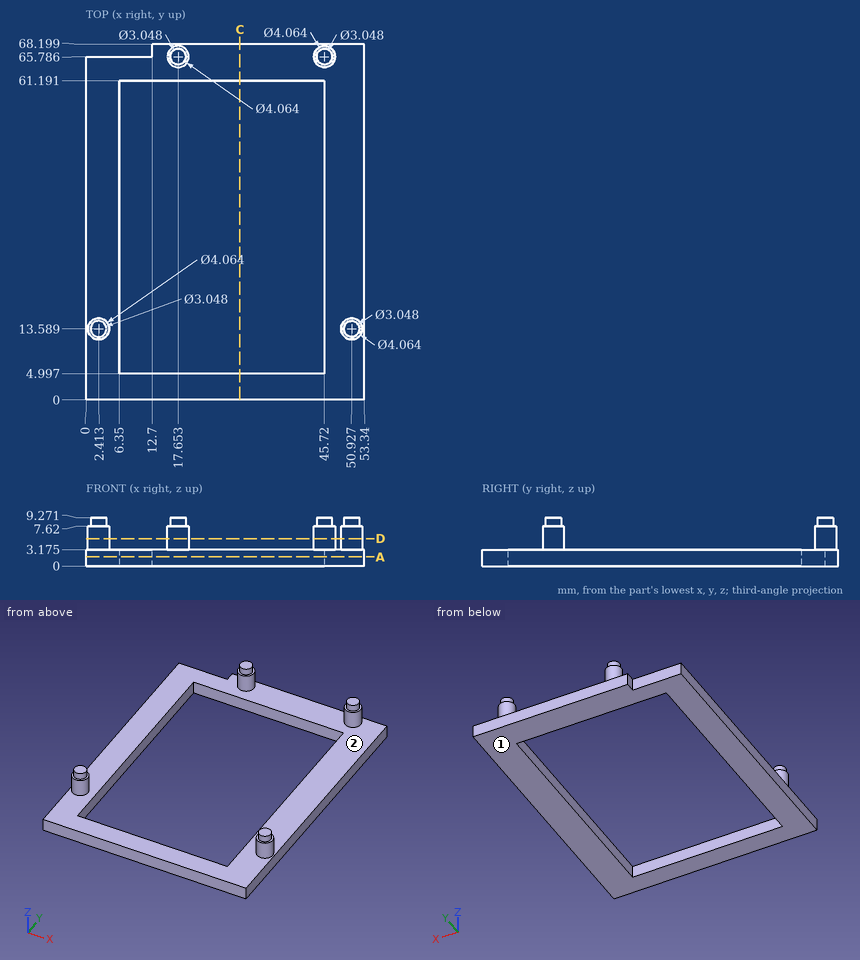
Geometry check sheet. Reference: drawing and pictorial views, mm from the part's lowest x, y, z. Give positions to 0.01 mm unless a question says otherwise; leave off trailing zeros. Order: outer loops, then holes, each group sorted by start corner. A loop starts at its lowest first (then second) coordinate and runs counter-clockwise, first axis right, second up.
1. Section check A-A, the plane z = 1.75. Enter the section's corners in (x, y).
2. Section check D-D, the plane z = 5.25. Enter the section's corners in (x, y) (1 decimal).
3. Section check C-C, the plane x = 29.5. Enter the section's corners in (y, z) (1 decimal), and give its area (3 significant figures).
4. Release check for a two-part mould opening along Z. For the marked faces 1 and 2 record: pulls with the +Z half, pulls with the -Z half, needs draft (parallel to the pull), parting line crosses it, or undercut.
5. Thickness scan on L1, parallel to X at y = 14.5, z = 2; L2, parallel to Y at x = 16, z = 1.5; L3, parallel to Z at x = 3, y = 16 (1 decimal). Record the ranges inside material, lowest first.
6. Gauge pin test, flat ends, axial feed: pin 1 Ø3.5 at (x, z) = (6.5, 2) entering from +Y; pin 2 Ø4 at (x, z) = (21.5, 2) entering from -Y; pin 3 Ø0.7 at (y, z) = (66.5, 1.5) entering from -X; pin 4 Ø10 at (x, y) = (39.5, 30.5) entering from +Z. Record the tip position at first contact, or that the pin passes through.
Values follow:
1. outline: (0, 0) - (53.34, 0) - (53.34, 68.2) - (12.7, 68.2) - (12.7, 65.79) - (0, 65.79) - close; hole (6.35, 5) - (45.72, 5) - (45.72, 61.19) - (6.35, 61.19) - close
2. outline: circle Ø4.1 at (2.4, 13.6); circle Ø4.1 at (17.7, 65.8); circle Ø4.1 at (45.7, 65.8); circle Ø4.1 at (50.9, 13.6)
3. outline: (0, 0) - (5, 0) - (5, 3.2) - (0, 3.2) - close; (61.2, 0) - (68.2, 0) - (68.2, 3.2) - (61.2, 3.2) - close
3. area: 38.1 mm2
4. face 1: pulls with the -Z half
4. face 2: pulls with the +Z half
5. L1: x = 0 to 6.35, 45.72 to 53.34
5. L2: y = 0 to 5, 61.19 to 68.2
5. L3: z = 0 to 3.2
6. pin 1: stops at y = 65.79
6. pin 2: stops at y = 0
6. pin 3: stops at x = 12.7
6. pin 4: passes through
